```python
from build123d import *

# Parameters (mm, degrees)
BOSS_EXTRUDE1_DEPTH   = 127
BOSS_EXTRUDE1_2_DEPTH = 127
BOSS_EXTRUDE1_3_DEPTH = 127
SKETCH3_R             = 355.614173825
BOSS_EXTRUDE2_DEPTH   = 6.35


with BuildPart() as part:
    # Sketch2 → Boss-Extrude1 (new body)
    with BuildSketch(Plane(origin=(0, 0, 0), x_dir=(1, 0, 0), z_dir=(0, 1, 0))):
        with BuildLine():
            ThreePointArc((-3.175, 355.6), (-307.970908478, 177.807086912), (-309.546133586, -175.050369343))
            Line((-309.546133586, -175.050369343), (-69.392656087, -36.397694462))
            ThreePointArc((-69.392656087, -36.397694462), (-67.860884615, 39.1795), (-3.175, 78.294650239))
            Line((-3.175, 78.294650239), (-3.175, 355.6))
        make_face()
    extrude(amount=BOSS_EXTRUDE1_DEPTH)



with BuildPart() as body_2:
    # Sketch2 → Boss-Extrude1 2 (new body)
    with BuildSketch(Plane(origin=(0, 0, 0), x_dir=(1, 0, 0), z_dir=(0, 1, 0))):
        with BuildLine():
            Line((69.392656087, -36.397694462), (309.546133586, -175.050369343))
            ThreePointArc((309.546133586, -175.050369343), (343.904371287, -90.505381247), (355.614173825, 0))
            ThreePointArc((355.614173825, 0), (252.577231384, 250.332144983), (3.175, 355.6))
            Line((3.175, 355.6), (3.175, 78.294650239))
            ThreePointArc((3.175, 78.294650239), (56.519566108, 54.274041014), (78.359, 0))
            ThreePointArc((78.359, 0), (76.084400567, -18.74291523), (69.392656087, -36.397694462))
        make_face()
    extrude(amount=BOSS_EXTRUDE1_2_DEPTH)


with BuildPart() as body_3:
    # Sketch2 → Boss-Extrude1 3 (new body)
    with BuildSketch(Plane(origin=(0, 0, 0), x_dir=(1, 0, 0), z_dir=(0, 1, 0))):
        with BuildLine():
            ThreePointArc((-306.371133586, -180.549630657), (0, -355.614173825), (306.371133586, -180.549630657))
            Line((306.371133586, -180.549630657), (66.217656087, -41.896955776))
            ThreePointArc((66.217656087, -41.896955776), (0, -78.359), (-66.217656087, -41.896955776))
            Line((-66.217656087, -41.896955776), (-306.371133586, -180.549630657))
        make_face()
    extrude(amount=BOSS_EXTRUDE1_3_DEPTH)


with BuildPart() as part_1:
    add(part.part)

    add(body_2.part)  # Boss-Extrude2 merges body 2

    add(body_3.part)  # Boss-Extrude2 merges body 3
    # Sketch3 → Boss-Extrude2 (add)
    with BuildSketch(Plane.XZ):
        Circle(SKETCH3_R)
    extrude(amount=BOSS_EXTRUDE2_DEPTH)


solid = part_1.part
```
Input: part model. Units: mm. Frame: model coordinates. A direction names the side the tool comes from. Round coordinates to 2 decimals unless told otherwise and drop trailing zeros. Loops run counter-clockwise (first coordinate to the right, second up) from the corner with the lowest first, then second, coordinate; pieces in that order, holes last.
1) Section query D-D on z = 139.5. Return the cut outline in (x, y).
Ans:
outline: (-327.11, -6.35) - (327.11, -6.35) - (327.11, 127) - (247.97, 127) - (247.97, 0) - (235.27, 0) - (235.27, 127) - (-235.27, 127) - (-235.27, 0) - (-247.97, 0) - (-247.97, 127) - (-327.11, 127) - close
2) Set-up query: faces 4 (the flat face through (3.175, 63, -219)), 5 (the flat face through (-184.61, 62.61, 110.25)), 6 (the flat face through (-5, -6.35, 5)). Return all of +Z, -Z, +X, -X, +Y, -Y with unobstructed straight access to the full face (end or side cutting, diameter ignored); none if empty.
Ans:
face 4: -Z, +Y
face 5: +Y
face 6: +Z, -Z, +X, -X, -Y
3) Material intervals for line 1 (X direction, y = 69, z = 118); line 2 (X direction, y = 88.5, z = -228) (3 decimals); line 3 (Z direction, x = 217.5, y = 17), sorted ascending.
Ans:
line 1: x = -335.47 to -210.73, -198.03 to 198.03, 210.73 to 335.47
line 2: x = -272.906 to -3.175, 3.175 to 272.906
line 3: z = -281.35 to 121.91, 129.24 to 281.35
4) Pin query (flat end, axial travel): pin 1 (6 mm diameter, centred on x = -161.5, y = 29, fed in from +Z); pin 2 (12 mm diameter, centred on x = 246, y = 62.5, fed in from -Z); pin 3 (1 mm diameter, centred on x = -141, y = 54.5, fed in from +Z). Return the tip coordinate at first contact, or that it passes through.
Ans:
pin 1: stops at z = 318.34
pin 2: stops at z = -262.41
pin 3: stops at z = 326.68
5) Section query A-A on y = 105. Return the cut outline in (x, z) (3 decimals).
Ans:
outline: (-309.546, 175.05) arc R355.614 ccw to (-3.175, -355.6) - (-3.175, -78.295) arc R78.359 cw to (-69.393, 36.398) - close; (-306.371, 180.55) - (-66.218, 41.897) arc R78.359 cw to (66.218, 41.897) - (306.371, 180.55) arc R355.614 ccw to start; (3.175, -355.6) arc R355.614 ccw to (309.546, 175.05) - (69.393, 36.398) arc R78.359 cw to (3.175, -78.295) - close
6) Section query B-B on z = -213.5. Return the cut outline in (x, y) (3 decimals), plus the area to 3 significant figures.
Ans:
outline: (-284.393, -6.35) - (284.393, -6.35) - (284.393, 127) - (3.175, 127) - (3.175, 0) - (-3.175, 0) - (-3.175, 127) - (-284.393, 127) - close
area: 75,000 mm2
7) Section query C-C on x = -137. Return the cut outline in (y, z), plus the area to 3 significant figures.
Ans:
outline: (-6.35, -328.17) - (127, -328.17) - (127, 75.43) - (0, 75.43) - (0, 82.76) - (127, 82.76) - (127, 328.17) - (-6.35, 328.17) - close
area: 86,600 mm2
8) Pull-direction query (X, two-part tool) for faces 1 (the cylindrical face through (1.1, 62.61, 78.35)), 2 (the flat face through (-4, 127, 197)), 3 (the cylindrical face through (-68.406, 62.611, -38.219)); classes: released by +X, released by -X, zero draft, split by the parting line, or undercut.
Ans:
face 1: undercut
face 2: zero draft
face 3: undercut
